Model file for the job. Use its own axes, mm. A direction names the side the tool comes from. Give positions to 0.01 mm unless a question says otherwise; leave off trailing zeros. Write each loop counter-clockwise with the first axis right and the second up, starting at its lowest first coordinate (ties: lowest second). Pieces come first, ordered by that corner, then holes. Notation, with made-up numbers: M 70.25,-2 L 127.25,-2 A30 cw 127.25,34 Z; hole C 44.5,-35 d11. An arc over 180 degrees is marked long. Answer as a JSON object with one key per item and string values. Group by question number.
Solid Edge part; units mm, degrees
sketch "Sketch1" plane through (0, 0, 0) normal (0, -1, 0) x (1, 0, 0)
  line L0 (-17.0509, 0) -> (-17.0509, 5)
  line L1 (-17.0509, 5) -> (17.9491, 5)
  line L2 (17.9491, 5) -> (17.9491, 0)
  line L3 (17.9491, 0) -> (27.9491, 0)
  line L4 (27.9491, 0) -> (27.9491, 15)
  line L5 (27.9491, 15) -> (-27.0509, 15)
  line L6 (-27.0509, 15) -> (-27.0509, 0)
  line L7 (-27.0509, 0) -> (-17.0509, 0)
extrude "Protrusion1" add sketch "Sketch1" along normal blind 50
extrude "ExtrudedCutout_3" [suppressed]
sketch "Sketch2" plane through (0, 0, 0) normal (1, 0, 0) x (0, 1, 0)
  line L0 (-50, 15) -> (-10, 15)
  line L1 (-10, 15) -> (-10, 50)
  line L2 (-10, 50) -> (-40, 50)
  arc A0 (-50, 35) -> (-40, 50) centre (-33.1234, 34.5823) cw
  line L3 (-50, 15) -> (-50, 35)
extrude "ExtrudedProtrusion_6" add sketch "Sketch2" along normal mid plane 15
sketch "Sketch3" plane through (7.5, -30, 32.5) normal (1, 0, 0) x (0, 1, 0)
  circle A0 centre (-10, 2.5) radius 5
extrude "ExtrudedCutout_4" cut sketch "Sketch3" against normal blind 55.8479
Q1. Drop flat-ended pins along their axis: P1, Ø2, axis at y = -26, z = 20, coming from the -X side; P2, Ø10, axis at x = -2, y = -42, coming from the -Z side; P3, Ø12, axis at x = -3.5, z = 38.5, coming from the +Y side. Give the stop position or say it passes through.
Q2. Slice it at B-B, the plane x = 5.5. Write the cut outline in (y, z), then the cut area to 3 significant figures.
Q3. Slice it at C-C, the plane y = -22.5. Write the cut outline in (x, z), then the cut area to 4 significant figures.
Q4. Slice it at D-D, the plane z = 44. Write the cut outline in (x, y), then the cut area to 3 significant figures.
Q5. Slice it at A-A, the plane y = -36. Write the cut outline in (x, z).
Q6. 3-axis set-ups, long thin cutter, end or side, ignore diameter. For faces 1 (the flat face through (0, -10, 32)), 2 (the flat face through (27.949, -25, 7)), 3 (the flat face through (7.5, -30, 32)), 4 (the flat face through (0, -25, 5)), 5 (the flat face through (1, 0, 9)): which of +Z, -Z, +X, -X, +Y, -Y reach the whole face in a straight line?
Q7. Two-plate mould, pull along X, no slides. Class faces 6 (the cylindrical face through (-0.11, -47.24, 43.84)), 7 (the flat face through (17.949, -25, 3)), 8 (the flat face through (-7.5, -30, 32)): +X half, -X half, draft (parallel to the pull), parting line (faces both ways), or undercut.
Q8. Wall check: L1, parallel to Z at x = -2, y = -40; L2, parallel to Z at x = 25.5, y = -1.5; L3, parallel to Y at x = -6, z = 29. Give the ranges that are in metal, low to high.
Solved:
{
 "1": {"P1": "stops at x = -7.5", "P2": "stops at z = 5", "P3": "stops at y = -10"},
 "2": {"outline": "M -50,5 L 0,5 L 0,15 L -10,15 L -10,50 L -40,50 A16.88 ccw -50,35 L -50,15 Z; hole C -40,35 d10", "area": "1,780 mm²"},
 "3": {"outline": "M -27.05,0 L -17.05,0 L -17.05,5 L 17.95,5 L 17.95,0 L 27.95,0 L 27.95,15 L 7.5,15 L 7.5,50 L -7.5,50 L -7.5,15 L -27.05,15 Z", "area": "1,175 mm²"},
 "4": {"outline": "M -7.5,-47.13 L 7.5,-47.13 L 7.5,-10 L -7.5,-10 Z", "area": "557 mm²"},
 "5": {"outline": "M -27.05,0 L -17.05,0 L -17.05,5 L 17.95,5 L 17.95,0 L 27.95,0 L 27.95,15 L 7.5,15 L 7.5,32 L -7.5,32 L -7.5,15 L -27.05,15 Z; M -7.5,38 L 7.5,38 L 7.5,50 L -7.5,50 Z"},
 "6": {"face 1": "+Z, +X, -X, +Y", "face 2": "+Z, -Z, +X, +Y, -Y", "face 3": "+Z, +X, +Y, -Y", "face 4": "-Z, +Y, -Y", "face 5": "+Z, -Z, +X, -X, +Y"},
 "7": {"face 6": "draft", "face 7": "undercut", "face 8": "-X half"},
 "8": {"L1": "z = 5 to 30, 40 to 50", "L2": "z = 0 to 15", "L3": "y = -50 to -10"}
}
